Read the model definition and answer for the solid it produces. Units are mm, in the model's axes. A direction names the side the tool comes from. Coordinates: 2 decimals unless noted, no trailing zeros. Order: outer loops, then holes, each group sorted by start corner. A loop starts at its lowest first (then second) coordinate and runs counter-clockwise, first axis right, second up. Notation, with made-up numbers: M -32.75,-34.75 L -23.75,-34.75 A26 cw -23.75,-2.75 Z; hole C 45.25,-16.75 d2. An arc over 180 degrees is marked long. Write each question's results on one line, items separated by ' | '.
```python
from build123d import *


with BuildPart() as f1:
    # F0 (on Front) → F1 (revolve)
    with BuildSketch(Plane.XZ):
        Polygon((-30, -41.6705080757), (-30, -43.6705080757), (0, -26.35), (10, -26.35), (10, -24.35), (2, -24.35), (2, -22.35), (0, -24.35), align=None)
    revolve(axis=Axis((-15, 0, 0), (-1, 0, 0)))

    # F0 (on Front) → F2 (revolve)
    with BuildSketch(Plane.XZ):
        Polygon((-30, -41.6705080757), (-30, -43.6705080757), (0, -26.35), (10, -26.35), (10, -24.35), (2, -24.35), (2, -22.35), (0, -24.35), align=None)
    revolve(axis=Axis((-15, 0, 0), (-1, 0, 0)))


solid = f1.part
```
(1) The part is cut by section A-A, the plane z = 0. Write down the section's boundary in (x, y).
Conclusion:
outline: M -30,-43.67 L 0,-26.35 L 10,-26.35 L 10,-24.35 L 2,-24.35 L 2,-22.35 L 0,-24.35 L -30,-41.67 Z; M -30,41.67 L 0,24.35 L 2,22.35 L 2,24.35 L 10,24.35 L 10,26.35 L 0,26.35 L -30,43.67 Z
(2) Given pin 1 (10 mm diameter, centred on x = -19, y = -13, fed in from -Z); pin 2 (1 mm diameter, centred on x = -18.5, z = 0, fed in from -Y); pin 3 (8 mm diameter, centred on x = -11.5, z = -2.5, fed in from -Y), each flat-ended and moving along its own axis, determine where each tip first touches the part or whether it passes through.
Conclusion:
pin 1: z = -38.42 | pin 2: y = -37.32 | pin 3: y = -35.22
(3) The part is cut by section D-D, the plane x = -8.5. Write down the section's boundary in (y, z).
Conclusion:
outline: C 0,0 d62.51; hole C 0,0 d58.51
(4) Straight lines are drawn through the part: line 1 (Y direction, x = 8.25, z = 0); line 2 (Y direction, x = -28, z = -18.5). For each, find the intervals that lie inside material, in ascending order.
Conclusion:
line 1: -26.35 to -24.35, 24.35 to 26.35 | line 2: -38.28 to -36.05, 36.05 to 38.28
(5) The part is cut by section C-C, the plane x = 6.5. Write down the section's boundary in (y, z).
Conclusion:
outline: C 0,0 d52.7; hole C 0,0 d48.7
(6) The mould has two halves that part along Y. Classify faces 1 (the conical face through (-1.457, 26.544, 5.894)), 2 (the flat face through (-30, 16, 39)), 3 (the cylindrical face through (5.94, 14.82, 19.32)): pulls with the +Y half, pulls with the -Y half, needs draft (parallel to the pull), parting line crosses it, or undercut.
Conclusion:
face 1: parting line crosses it | face 2: needs draft | face 3: undercut
(7) For faces 4 (the flat face through (2, 20, -11)), 5 (the flat face through (10, 23.3, -7.7)), determine the directions among +Z, -Z, +X, -X, +Y, -Y from which every point of the face is accessible in a straight line to the end or side of a thin tool.
Conclusion:
face 4: +X | face 5: +Z, -Z, +X, +Y, -Y
